Input: part model. Units: mm. Frame: model coordinates. A direction names the side the tool comes from. Coordinates: 2 decimals unless noted, no trailing zeros. Order: outer loops, then holes, each group sorted by start corner. A loop starts at its lowest first (then second) coordinate and runs counter-clockwise, first axis right, second up. Notation, with made-up numbers: (15.5, 73.25) -> (43.5, 73.25) arc R23 cw to (43.5, 109.25) -> close; hole circle Ø4 at (42.5, 81.5). An arc over 180 degrees is marked (long way). One line per question, with ' | ' between items.
```python
from build123d import *

# Parameters (mm, degrees)
F1_DEPTH = 12.7
F2_W     = 67.693748
F2_H     = 67.693748
F3_DEPTH = 12.7
F5_DEPTH = 12.7
F7_DEPTH = 12.7


with BuildPart() as f1:
    # F0 (on Top) → F1 (new body)
    with BuildSketch(Plane.XY):
        Polygon((0, 14.688266), (12.772406, 0), (67.693748, 0), (67.693748, 67.693748), (0, 67.693748), align=None)
    extrude(amount=F1_DEPTH)

    # F2 (on face) → F3 (join)
    with BuildSketch(Plane.XY.offset(12.7)):
        with Locations((33.846874, 33.846874)):
            Rectangle(F2_W, F2_H)
    extrude(amount=F3_DEPTH)

    # F4 (on face) → F5 (join)
    with BuildSketch(Plane.XY.offset(25.4)):
        Polygon((67.693748, 67.693748), (0, 67.693748), (0, 18.519988), (11.860092, 18.519988), (11.860092, 10.674083), (19.888459, 10.674083), (19.888459, 0), (67.693748, 0), align=None)
    extrude(amount=F5_DEPTH)

    # F6 (on face) → F7 (join)
    with BuildSketch(Plane.XY.offset(38.1)):
        Polygon((18.210092, 17.024082), (26.238458, 17.024082), (26.238458, 0), (67.693748, 0), (67.693748, 67.693748), (0, 67.693748), (0, 24.869988), (18.210092, 24.869988), align=None)
    extrude(amount=F7_DEPTH)


solid = f1.part
```
1. Ray query, line 1 (X direction, y = 5.5, z = 37); line 2 (Z direction, x = 15.5, y = 3.5); line 3 (Y direction, x = 22, z = 46.5). Return the intervals inside material, ascending. Write a range as [from, to].
Recorded:
line 1: x = [19.89, 67.69] | line 2: z = [0, 25.4] | line 3: y = [17.02, 67.69]
2. Cut plane B-B, the plane y = 6. Return loops of the section in (x, z).
Recorded:
outline: (0, 12.7) -> (7.56, 12.7) -> (7.56, 0) -> (67.69, 0) -> (67.69, 50.8) -> (26.24, 50.8) -> (26.24, 38.1) -> (19.89, 38.1) -> (19.89, 25.4) -> (0, 25.4) -> close
3. Pin query (flat end, axial travel): pin 1 Ø13 at (x, z) = (6.5, 30.5) entering from -Y; pin 2 Ø11.5 at (y, z) = (4, 33) entering from -X; pin 3 Ø2.5 at (y, z) = (15, 33.5) entering from -X; pin 4 Ø2.5 at (y, z) = (21, 46.5) entering from -X. Return the tip coordinate at first contact, or that it passes through.
Recorded:
pin 1: stops at y = 0 | pin 2: stops at x = 19.89 | pin 3: stops at x = 11.86 | pin 4: stops at x = 18.21
4. Cut plane A-A, the plane z = 39. Return loops of the section in (x, y), and give its area (3 significant figures).
Recorded:
outline: (0, 24.87) -> (18.21, 24.87) -> (18.21, 17.02) -> (26.24, 17.02) -> (26.24, 0) -> (67.69, 0) -> (67.69, 67.69) -> (0, 67.69) -> close | area: 3,990 mm^2
5. Cut plane C-C, the plane z = 4. Return loops of the section in (x, y), and give its area (3 significant figures).
Recorded:
outline: (0, 14.69) -> (12.77, 0) -> (67.69, 0) -> (67.69, 67.69) -> (0, 67.69) -> close | area: 4,490 mm^2
6. Access query for faces 1 (the face through (0, 42, 25)), 2 (the face through (26.238, 9, 44)), 3 (the face through (6.297, 7.447, 6.261)). Directions: +Z, -Z, +X, -X, +Y, -Y. A direction counts if a zero-diameter tool reaches every point of the face in a straight line with its end or side. Return the directions, or none.
Recorded:
face 1: +Z, -Z, -X, +Y, -Y | face 2: +Z, -X, -Y | face 3: -Z, -X, -Y
